Could you check a few things on this model? Use its own coordinates, in mm. A direction names the side the tool comes from. Coordinates: 2 decimals unless noted, no trailing zeros. Loops run counter-clockwise (first coordinate to the right, second up) from the corner with the lowest first, then second, coordinate; pieces in that order, holes last. Notation, with made-up numbers: M 43.25,27 L 75.25,27 A18 cw 75.25,32 Z; hole C 54,-21 d4. An arc over 180 degrees is marked long. Use one line per item in the form item = value. Start each with the question number.
```python
from build123d import *
from OCP.BRepAlgoAPI import BRepAlgoAPI_Cut
from OCP.TopTools import TopTools_ListOfShape

# Parameters (mm, degrees)
SKETCH2_R           = 5.5
SKETCH2_R_2         = 1
BOSS_EXTRUDE1_DEPTH = 10
SCALE1_SCALE        = 0.9
SKETCH3_R           = 2.8
CUT_EXTRUDE1_DEPTH  = 3
SKETCH4_R           = 1.42
CUT_EXTRUDE2_DEPTH  = 7
SKETCH6_R           = 12.614646558
SKETCH6_R_2         = 9
CUT_EXTRUDE3_DEPTH  = 10


with BuildPart() as part:
    # Sketch1 → Revolve1 (revolve)
    with BuildSketch(Plane.XY, mode=Mode.PRIVATE) as revolve1_sk:
        with BuildLine():
            Line((-7, 9), (5, 9))
            add(Edge.make_bspline(
                [(5, 9), (5, 8.856466181), (4.980630385, 8.552638111), (4.879856885, 8.085906437), (4.637540593, 7.528306389), (3.996049584, 6.69016035), (2.86097235, 5.618747783), (1.478465211, 4.503997435), (0.514957064, 3.794701588), (0.068439653, 3.476275963), (0, 3.427716912)],
                knots=[0, 0, 0, 0, 0.0625, 0.125, 0.25, 0.375, 0.5, 0.625, 0.75, 0.773497894, 0.773497894, 0.773497894, 0.773497894], degree=3))
            Line((0, 3.427716912), (0, 1))
            add(Edge.make_bspline(
                [(7, 9), (7, 7.437991686), (5.451200792, 4.581787455), (0.00160793, 1.001387392), (0, 1)],
                knots=[0, 0, 0, 0, 0.405901642, 1, 1, 1, 1], degree=3))
            Line((7, 9), (7, 11))
            Line((7, 11), (6, 11))
            Line((6, 11), (6, 10.9))
            ThreePointArc((6, 10.9), (5.736396103, 10.263603897), (5.1, 10))
            Line((5.1, 10), (-5.1, 10))
            ThreePointArc((-5.1, 10), (-5.736396103, 10.263603897), (-6, 10.9))
            Line((-6, 10.9), (-6, 11))
            Line((-6, 11), (-7, 11))
            Line((-7, 11), (-7, 9))
        make_face()
    revolve(revolve1_sk.sketch.rotate(Axis((0, 0, 0), (1, 0, 0)), 90), axis=Axis((0, 0, 0), (1, 0, 0)))

    # Sketch2 → Boss-Extrude1 (add)
    with BuildSketch(Plane.ZY.offset(7)):
        Circle(SKETCH2_R)
        Circle(SKETCH2_R_2, mode=Mode.SUBTRACT)
    extrude(amount=-BOSS_EXTRUDE1_DEPTH)


with BuildPart() as part_1:
    # Scale1: scaled about (0.211743698, 3.8e-08, 1.4215e-05)
    add(part.part.scale(SCALE1_SCALE).moved(Location((0.02117437, 4e-09, 1.421e-06))))

    # Sketch3 → Cut-Extrude1 (cut)
    with BuildSketch(Plane(origin=(2.721175281, 0, 0), x_dir=(0, 0, -1), z_dir=(1, 0, 0))):
        Circle(SKETCH3_R)
    extrude(amount=-CUT_EXTRUDE1_DEPTH, mode=Mode.SUBTRACT)


with BuildPart() as cut_extrude2_tool:
    # Sketch4 → Cut-Extrude2 (new body)
    with BuildSketch(Plane.ZY.offset(6.278824719)):
        with Locations((-8.53e-07, 0)):
            Circle(SKETCH4_R)
    extrude(amount=-CUT_EXTRUDE2_DEPTH)


with BuildPart() as part_2:
    add(part_1.part)

    # Cut-Extrude2: cut by cut_extrude2_tool, with a tolerance
    cut_extrude2_stock = TopTools_ListOfShape()
    cut_extrude2_stock.Append(part_2.part.wrapped)
    cut_extrude2_tools = TopTools_ListOfShape()
    cut_extrude2_tools.Append(cut_extrude2_tool.part.wrapped)
    cut_extrude2_cut = BRepAlgoAPI_Cut()
    cut_extrude2_cut.SetArguments(cut_extrude2_stock)
    cut_extrude2_cut.SetTools(cut_extrude2_tools)
    cut_extrude2_cut.SetFuzzyValue(0.00001)
    cut_extrude2_cut.Build()
    add(Compound.cast(cut_extrude2_cut.Shape()).solids(), mode=Mode.REPLACE)


with BuildPart() as cut_extrude3_tool:
    # Sketch6 → Cut-Extrude3 (new body)
    with BuildSketch(Plane(origin=(0, 0, 0), x_dir=(0, 0, -1), z_dir=(1, 0, 0))):
        with Locations((8.53e-07, 0)):
            Circle(SKETCH6_R)
        with Locations(Location((8.53e-07, 0, 0), (0, 0, 180))):
            Circle(SKETCH6_R_2, mode=Mode.SUBTRACT)
    extrude(amount=-CUT_EXTRUDE3_DEPTH)


with BuildPart() as part_3:
    add(part_2.part)

    # Cut-Extrude3: cut by cut_extrude3_tool, with a tolerance
    cut_extrude3_stock = TopTools_ListOfShape()
    cut_extrude3_stock.Append(part_3.part.wrapped)
    cut_extrude3_tools = TopTools_ListOfShape()
    cut_extrude3_tools.Append(cut_extrude3_tool.part.wrapped)
    cut_extrude3_cut = BRepAlgoAPI_Cut()
    cut_extrude3_cut.SetArguments(cut_extrude3_stock)
    cut_extrude3_cut.SetTools(cut_extrude3_tools)
    cut_extrude3_cut.SetFuzzyValue(0.00001)
    cut_extrude3_cut.Build()
    add(Compound.cast(cut_extrude3_cut.Shape()).solids(), mode=Mode.REPLACE)


solid = part_3.part
```
Item 1: For faces 4 (the flat face through (-0.279, -1.2, -1.2)), 5 (the cylindrical face through (-0.803, -2.433, 7.726)), 6 (the flat face through (6.321, -1.513, 8.113)), which set-ups out of +Z, -Z, +X, -X, +Y, -Y let a thin tool reach every point of the face, with its end or its side?
Item 2: Thinking about a two-plate mould opening in Z: for faces 1 (the cylindrical face through (5.865, -9.816, -1.289)), 2 (the cylindrical face through (-3.32, 0.06, -1.42)), 3 (the flat face through (-6.279, 1.2, -1.2)), which applies, pulls with the +Z half, pulls with the -Z half, needs draft (parallel to the pull), parting line crosses it, or undercut?
Item 3: I want a section at B-B (x = -2). Write out the boundary of the cut face in (y, z).
Item 4: I'm going to push flat-ended pins straight in: P1, Ø5, axis at x = -5, y = -6, coming from the +Z side; P2, Ø2, axis at y = 1, z = -2, coming from the +X side; P3, Ø5, axis at x = -1.5, y = 0.5, coming from the -Z side. Where does each tip first touch, or does it pass through?
Item 5: I want a section at A-A (x = 0). Write out the boundary of the cut face in (y, z), plus the area to 3 significant figures.
Item 6: Please list where these lines run through material, in increasing order: line 1 along Y through (x, z) = (1.5, 0); line 2 along Y through (x, z) = (-1.8, 0); line 3 along Z through (x, y) = (-1.5, -2.5).
Worked answers:
q1.face_4 = +X
q1.face_5 = -X
q1.face_6 = +Z, -Z, +X, +Y, -Y
q2.face_1 = parting line crosses it
q2.face_2 = undercut
q2.face_3 = needs draft
q3.outline = C 0,0 d18; C 0,0 d9.9; hole C 0,0 d16.2; hole C 0,0 d2.84
q4.P1 = 8.29
q4.P2 = 3.2
q4.P3 = -9
q5.outline = C 0,0 d18; C 0,0 d9.9; hole C 0,0 d16.2; hole C 0,0 d5.6
q5.area = 101 mm²
q6.line_1 = -9 to -8.1, -4.95 to -2.8, 2.8 to 4.95, 8.1 to 9
q6.line_2 = -9 to -8.1, -4.95 to -1.42, 1.42 to 4.95, 8.1 to 9
q6.line_3 = -8.65 to -7.7, -4.27 to 4.27, 7.7 to 8.65
